Read the model definition and answer for the solid it produces. Units are mm, in the model's axes. A direction names the side the tool comes from. Coordinates: 2 decimals unless noted, no trailing zeros. Loops run counter-clockwise (first coordinate to the right, second up) from the corner with the lowest first, then second, coordinate; pieces in that order, holes last. Notation, with made-up numbers: (48.25, -21.75) - (76.25, -21.75) arc R22 cw to (76.25, 14.25) - close; hole circle Ø10 at (-16, 2.5). An arc over 180 degrees is marked (long way). One line per item, written item: value. Start each with the question number.
from build123d import *

# Parameters (mm, degrees)
BOSS_EXTRUDE1_DEPTH      = 4.875
BOSS_EXTRUDE1_DEPTH_BACK = 4.875
SKETCH3_R                = 1.2
CUT_EXTRUDE1_DEPTH       = 6.161940042
FILLET1_R                = 0.078539816
CIRPATTERN1_COUNT        = 10
FILLET1_OF_CIRPATTERN1_R = 0.078539816


with BuildPart() as part:
    # Sketch3 → Boss-Extrude1 (new, two sides: drawn at the far end of the back side and taken through both)
    with BuildSketch(Plane.XY.offset(-BOSS_EXTRUDE1_DEPTH_BACK)):
        Circle(SKETCH3_R)
    extrude(amount=BOSS_EXTRUDE1_DEPTH + BOSS_EXTRUDE1_DEPTH_BACK)

    # Sketch4 → Cut-Extrude1 (cut, symmetric)
    with BuildSketch(Plane.XY):
        with BuildLine():
            Line((0.796135351, -0.078539816), (0.796135351, 0.078539816))
            ThreePointArc((0.796135351, 0.078539816), (0.998479062, 0.163721965), (1.158053404, 0.314503282))
            ThreePointArc((1.158053404, 0.314503282), (1.2, 0), (1.158053404, -0.314503282))
            ThreePointArc((1.158053404, -0.314503282), (0.998479062, -0.163721965), (0.796135351, -0.078539816))
        make_face()
    cut_extrude1 = extrude(amount=CUT_EXTRUDE1_DEPTH, both=True, mode=Mode.SUBTRACT)

    # Fillet1
    fillet1_edges = [part.edges().sort_by_distance(p)[0] for p in [
        (0.796135351, 0.078539816, 0),
        (0.796135351, -0.078539816, 0),
    ]]
    fillet(fillet1_edges, radius=FILLET1_R)

    # CirPattern1: Cut-Extrude1 ×10 about axis
    cirpattern1_axis = Axis((0, 0, 0), (0, 0, 1))
    for i in range(1, CIRPATTERN1_COUNT):
        add(cut_extrude1.rotate(cirpattern1_axis, i * 360 / CIRPATTERN1_COUNT), mode=Mode.SUBTRACT)

    # Fillet1 of CirPattern1
    fillet1_of_cirpattern1_edges = [part.edges().sort_by_distance(p)[0] for p in [
        (0.597922483, 0.531496664, 0),
        (0.690251575, 0.404416572, 0),
        (0.171323549, 0.781439851, 0),
        (0.320715157, 0.732899576, 0),
        (-0.320715157, 0.732899576, 0),
        (-0.171323549, 0.781439851, 0),
        (-0.690251575, 0.404416572, 0),
        (-0.597922483, 0.531496664, 0),
        (-0.796135351, -0.078539816, 0),
        (-0.796135351, 0.078539816, 0),
        (-0.597922483, -0.531496664, 0),
        (-0.690251575, -0.404416572, 0),
        (-0.171323549, -0.781439851, 0),
        (-0.320715157, -0.732899576, 0),
        (0.320715157, -0.732899576, 0),
        (0.171323549, -0.781439851, 0),
        (0.690251575, -0.404416572, 0),
        (0.597922483, -0.531496664, 0),
    ]]
    fillet(fillet1_of_cirpattern1_edges, radius=FILLET1_OF_CIRPATTERN1_R)

    # Sketch6 → Cut-Revolve1 (revolve, cut)
    with BuildSketch(Plane(origin=(0, 0, 0), x_dir=(1, 0, 0), z_dir=(0, 1, 0))):
        Polygon((-0.44, 4.875), (-1.3, 4.875), (-1.3, -1.125), (-0.75, -1.125), (-0.75, 3.925), (-0.44, 3.925), align=None)
        Polygon((-1.3, -2.625), (-1.3, -4.875), (-0.44, -4.875), (-0.44, -3.925), (-1.025, -3.925), (-1.025, -2.625), align=None)
    revolve(axis=Axis((0, 0, -6.2826103), (0, 0, 1)), mode=Mode.SUBTRACT)


solid = part.part
1) Straight lines are drawn through the part: L1, parallel to Y at x = -0.1, z = -3; L2, parallel to Z at x = 0.7, y = 0 (3 decimals); L3, parallel to Z at x = 1, y = -0.4 (3 decimals). For each, find the intervals that lie inside material, in ascending order.
2) Flat-ended cylindrical pins translate along their axes: P1, Ø1, axis at y = 0, z = -3, coming from the +X side; P2, Ø1, axis at x = -1, y = 0, coming from the -Z side (3 decimals). Find the tip coordinate at first contact, or state that the pin passes through.
3) For faces 1 (the flat face through (0, 0, 4.875)), 2 (the cylindrical face through (0.1, 0.43, 4.39)), 3 (the cylindrical face through (0.75, -0.03, -1.44)), determine the directions among +Z, -Z, +X, -X, +Y, -Y from which every point of the face is accessible in a straight line to the end or side of a thin tool.
4) Section A-A, the plane z = -1.25 is taken. Determine the outline of the cut face in (x, y).
Answer below:
1. L1: -0.74 to 0.74
1. L2: -3.925 to 3.925
1. L3: 1.125 to 2.625
2. P1: x = 0.75
2. P2: z = -3.925
3. face 1: +Z, +X, -X, +Y, -Y
3. face 2: +Z
3. face 3: -Z
4. outline: circle Ø1.5 at (0, 0)
